Source: CAD feature listing. Evaluate the final solid. Frame: model axes, mm. Give positions to 0.01 mm unless a question says otherwise; leave off trailing zeros. Loops run counter-clockwise (first coordinate to the right, second up) from the corner with the lowest first, then second, coordinate; pieces in that order, holes last.
```python
from build123d import *
from build123d.topology import SkipClean

# Parameters (mm, degrees)
EXTRUDE_1_DEPTH     = 3.96
SKETCH_3_R          = 1.25
CUT_EXTRUDE_1_DEPTH = 2
CUT_EXTRUDE_2_DEPTH = 0.5
SKETCH_5_R          = 0.4
EXTRUDE_2_DEPTH     = 5


with BuildPart() as part:
    # 草图1 → 凸台-拉伸1 (new body)
    with BuildSketch(Plane(origin=(0, 0, 0), x_dir=(0, 0, -1), z_dir=(1, 0, 0))):
        Polygon((3.4, 0), (-3.4, 0), (-3.4, 4.5), (-2, 8.5), (2, 8.5), (3.4, 4.5), align=None)
    extrude(amount=EXTRUDE_1_DEPTH)

    # 草图3 → 切除-拉伸1 (cut)
    with BuildSketch(Plane(origin=(0, 8.5, 0), x_dir=(1, 0, 0), z_dir=(0, 1, 0))):
        with Locations(Location((1.98, 0, 0), (0, 0, 270))):
            Circle(SKETCH_3_R)
    extrude(amount=-CUT_EXTRUDE_1_DEPTH, mode=Mode.SUBTRACT)

    # 草图4 → 切除-拉伸2 (cut)
    with SkipClean():  # the faces are left unmerged after this step: merging them gives an invalid solid
        with BuildSketch(Plane(origin=(0, 6.5, 0), x_dir=(1, 0, 0), z_dir=(0, 1, 0))):
            with BuildLine():
                Line((0.755255129, 0.25), (3.204744871, 0.25))
                ThreePointArc((3.204744871, 0.25), (3.23, 0), (3.204744871, -0.25))
                Line((3.204744871, -0.25), (0.755255129, -0.25))
                ThreePointArc((0.755255129, -0.25), (0.73, 0), (0.755255129, 0.25))
            make_face()
        extrude(amount=-CUT_EXTRUDE_2_DEPTH, mode=Mode.SUBTRACT)

    # 草图5 → 凸台-拉伸2 (add)
    with SkipClean():  # the faces are left unmerged after this step: merging them gives an invalid solid
        with BuildSketch(Plane.XZ):
            with Locations(Location((1.98, 0, 0), (0, 0, 90))):
                Circle(SKETCH_5_R)
        extrude(amount=EXTRUDE_2_DEPTH)


solid = part.part
```
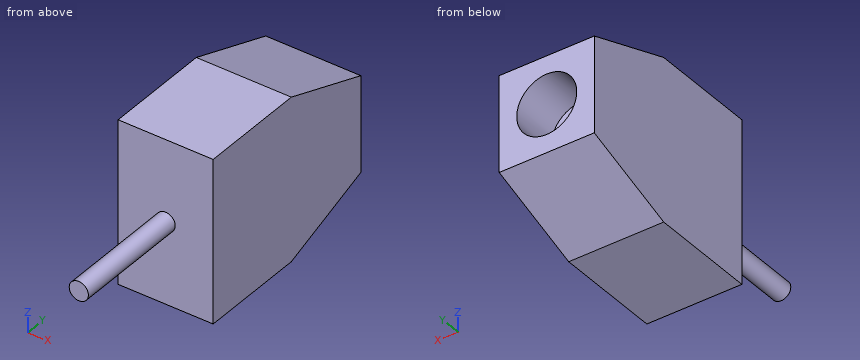
(1) Section D-D, the plane y = -0.5. Return the cut outline in (x, z).
A:
outline: circle Ø0.8 at (1.98, 0)
(2) Section C-C, the plane z = -0.75. Return the cut outline in (x, y).
A:
outline: (0, 0) - (3.96, 0) - (3.96, 8.5) - (2.98, 8.5) - (2.98, 6.5) - (0.98, 6.5) - (0.98, 8.5) - (0, 8.5) - close
(3) Section A-A, the plane x = 1.98. Return the cut outline in (y, z), then the cut area to 4 significant figures.
A:
outline: (-5, -0.4) - (0, -0.4) - (0, -3.4) - (4.5, -3.4) - (8.5, -2) - (8.5, -1.25) - (6.5, -1.25) - (6.5, -0.25) - (6, -0.25) - (6, 0.25) - (6.5, 0.25) - (6.5, 1.25) - (8.5, 1.25) - (8.5, 2) - (4.5, 3.4) - (0, 3.4) - (0, 0.4) - (-5, 0.4) - close
area: 50.95 mm2
(4) First-contact query: pin 1 (0.5 mm diameter, centred on x = 1.5, z = -0.5, fed in from +Y). Flat tip, straight axial feed; report the tip coordinate or a pass-through.
A:
pin 1: stops at y = 6.5
(5) Ray query, line 1 along X through (y, z) = (7.5, -0.25); line 2 along Y through (x, z) = (1.85, 0.75); line 3 along Y through (x, z) = (3.75, -1). Return the intervals inside material, ascending.
A:
line 1: x = 0 to 0.76, 3.2 to 3.96
line 2: y = 0 to 6.5
line 3: y = 0 to 8.5
